Input: part model. Units: mm. Frame: model coordinates. Face numbers are marked on the shaded views. A direction names the side the tool comes from. Round coordinates to 2 decimals unless told otherwise and drop trailing zeros. Loops run counter-clockwise (first coordinate to the right, second up) from the corner with the lowest first, then second, coordinate; pieces in that order, holes last.
1) Section C-C, the plane y = 2.5. Return loops of the section in (x, z).
2) Section A-A, the plane z = 5.75. Return loops of the section in (x, y), and give its area (3 significant figures).
3) First-contact query: pin 1 (3 mm diameter, centred on y = -1.5, z = 10.5, fed in from +X); pin 2 (7.5 mm diameter, centred on x = 1, y = 8.5, fed in from +Z); pin 3 (1 mm diameter, centred on y = 13, z = 13, fed in from +X). Flat tips, straight axial feed; report the tip coordinate or a pass-through.
4) Draft query along X for the marked faces 1, 2, 3 and 4. Return one class per face: pulls with the +X half, pulls with the -X half, needs draft (parallel to the pull), parting line crosses it, or undercut.
5) Ray query, line 1 along Y through (x, z) = (-6.25, 11.25); line 2 along X through (y, z) = (-8.25, 2.15); line 3 along X through (y, z) = (-8.25, -1.2). Return the intervals inside material, ascending.
6) Section B-B, the plane x = 0. Return loops of the section in (y, z).
7) Access query for the marked faces 5, 6 and 7. Directions: +Z, -Z, +X, -X, +Y, -Y. A direction counts if a zero-diameter tool reaches every point of the face in a straight line with its end or side. Return the directions, or none.
from build123d import *

# Parameters (mm, degrees)
F4_DEPTH       = 13.5
F4_DEPTH_BACK  = 3
F5_R           = 4
F6_T           = -1.2
F7_W           = 6.6
F7_H           = 6
F8_DEPTH       = 13.75
F8_DEPTH_BACK  = 13.75
F3_W           = 8
F3_H           = 8.5
F9_DEPTH       = 4.5
F9_DEPTH_BACK  = 4.3
F11_START      = -6.5
F10_W          = 10.5
F10_H          = 18.4398862173
F11_DEPTH      = 11.4
F12_F1_R       = 4
F12_F2_R       = 4
F12_F3_R       = 4
F12_F4_R       = 4
F0_R           = 1.25
F13_DEPTH      = 7.9
F13_DEPTH_BACK = 7.1
F1_R           = 2.5
F14_DEPTH      = 1.8
F14_DEPTH_BACK = 4.3
F15_R          = 5
F17_DEPTH      = 16
F17_DEPTH_BACK = 16.1
F18_W          = 5.6
F18_H          = 3
F19_DEPTH      = 25
F19_DEPTH_BACK = 25


# Not quite as in the source:
# - a feature names something its author has since deleted; it is built from what else it names


with BuildPart() as f4:
    # F2 (on Top) → F4 (new body, two sides)
    with BuildSketch(Plane.XY) as f4_sk:
        with BuildLine():
            Line((2.6, 4.25), (2.6, 13.75))
            Line((2.6, 13.75), (-16, 13.75))
            Line((-16, 13.75), (-16, -13.75))
            Line((-16, -13.75), (2.6, -13.75))
            Line((2.6, -13.75), (2.6, -4.25))
            Line((2.6, -4.25), (-4.5505102572, -4.25))
            ThreePointArc((-4.5505102572, -4.25), (-8.769806787, -4.7695668459), (-10.3781091101, -0.8343697034))
            Line((-10.3781091101, -0.8343697034), (-9, 4.25))
            Line((-9, 4.25), (2.6, 4.25))
        make_face()
    extrude(amount=F4_DEPTH)
    extrude(f4_sk.sketch, amount=-F4_DEPTH_BACK)

    # F5
    f5_edges = [f4.edges().sort_by_distance(p)[0] for p in [
        (-16, 13.75, 5.25),
        (-16, -13.75, 5.25),
    ]]
    fillet(f5_edges, radius=F5_R)

    # F6
    f6_openings = [f4.faces().sort_by_distance(p)[0] for p in [
        (-4.7, 13.418005, 13.5),
        (2.6, 9, 5.25),
        (2.6, -9, 5.25),
        (-0.975255, -4.25, 5.25),
        (-3.2, 4.25, 5.25),
        (-8.769807, -4.769567, 5.25),
        (-9.689055, 1.707815, 5.25),
    ]]
    offset(amount=F6_T, openings=f6_openings)

    # F7 (on Front) → F8 (join, two sides)
    with BuildSketch(Plane.XZ) as f8_sk:
        with Locations((-0.7, 0)):
            Rectangle(F7_W, F7_H)
    extrude(amount=-F8_DEPTH)
    extrude(f8_sk.sketch, amount=F8_DEPTH_BACK)

    # F3 (on Top) → F9 (cut, two sides)
    with BuildSketch(Plane.XY) as f9_sk:
        with Locations((-1.4, 0)):
            Rectangle(F3_W, F3_H)
    extrude(amount=F9_DEPTH, mode=Mode.SUBTRACT)
    extrude(f9_sk.sketch, amount=-F9_DEPTH_BACK, mode=Mode.SUBTRACT)

    # F10 (on Right) → F11 (cut)
    with BuildSketch(Plane.YZ.offset(F11_START)):
        with Locations((2.5, 10.7199431086)):
            Rectangle(F10_W, F10_H)
    extrude(amount=-F11_DEPTH, mode=Mode.SUBTRACT)

    # F12: fillet of radius 4 on 4 edges, made by hand

    # F12_f1
    f12_f1_edges = [f4.edges().sort_by_distance(p)[0] for p in [
        (-4, -4.25, 0.6),
    ]]
    fillet(f12_f1_edges, radius=F12_F1_R)

    # F12_f2
    f12_f2_edges = [f4.edges().sort_by_distance(p)[0] for p in [
        (-4, 4.25, 0.6),
    ]]
    fillet(f12_f2_edges, radius=F12_F2_R)

    # F12_f3
    f12_f3_edges = [f4.edges().sort_by_distance(p)[0] for p in [
        (2.6, 4.25, 0),
    ]]
    fillet(f12_f3_edges, radius=F12_F3_R)

    # F12_f4
    f12_f4_edges = [f4.edges().sort_by_distance(p)[0] for p in [
        (2.6, -4.25, 0),
    ]]
    fillet(f12_f4_edges, radius=F12_F4_R)

    # F0 (on Top) → F13 (cut, two sides)
    with BuildSketch(Plane.XY) as f13_sk:
        with Locations((0, -8.25)):
            Circle(F0_R)
        with Locations((0, 8.25)):
            Circle(F0_R)
    extrude(amount=F13_DEPTH, mode=Mode.SUBTRACT)
    extrude(f13_sk.sketch, amount=-F13_DEPTH_BACK, mode=Mode.SUBTRACT)

    # F1 (on Top) → F14 (cut, two sides)
    with BuildSketch(Plane.XY) as f14_sk:
        with Locations((0, -8.25)):
            Circle(F1_R)
        with Locations((0, 8.25)):
            Circle(F1_R)
    extrude(amount=F14_DEPTH, mode=Mode.SUBTRACT)
    extrude(f14_sk.sketch, amount=-F14_DEPTH_BACK, mode=Mode.SUBTRACT)

    # F15
    f15_edges = [f4.edges().sort_by_distance(p)[0] for p in [
        (-4.55051, -4.25, -2.4),
        (-9, 4.25, -2.4),
    ]]
    fillet(f15_edges, radius=F15_R)

    # F16 (on Front) → F17 (cut, two sides)
    with BuildSketch(Plane.XZ) as f17_sk:
        Polygon((2.6, 1.8), (-4.0077234488, -6.074778159), (2.3954068281, -10.9375437775), (8.7053719483, -6.2603745918), align=None)
    extrude(amount=F17_DEPTH, mode=Mode.SUBTRACT)
    extrude(f17_sk.sketch, amount=-F17_DEPTH_BACK, mode=Mode.SUBTRACT)

    # F18 (on Front) → F19 (cut, two sides)
    with BuildSketch(Plane.XZ) as f19_sk:
        with Locations((-0.2, 13.5)):
            Rectangle(F18_W, F18_H)
    extrude(amount=F19_DEPTH, mode=Mode.SUBTRACT)
    extrude(f19_sk.sketch, amount=-F19_DEPTH_BACK, mode=Mode.SUBTRACT)


solid = f4.part
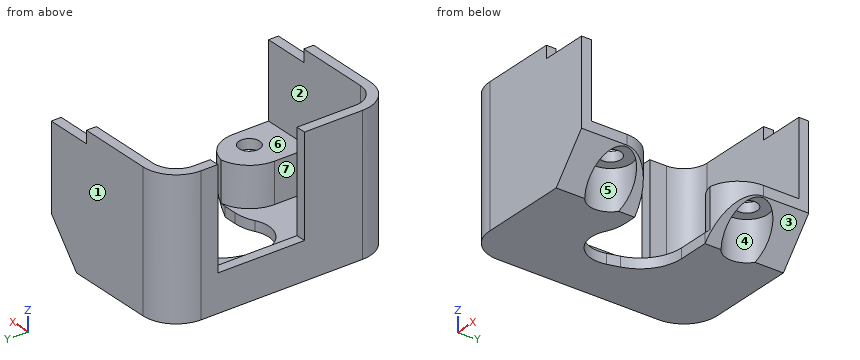
Final values:
1. outline: (-16, -3) - (-8.97, -3) - (-8.97, -1.8) - (-14.8, -1.8) - (-14.8, 1.5) - (-16, 1.5) - close
2. outline: (-16, -9.75) arc R4 ccw to (-12, -13.75) - (2.6, -13.75) - (2.6, -12.55) - (-12, -12.55) arc R2.8 cw to (-14.8, -9.75) - (-14.8, -2.75) - (-16, -2.75) - close; (-16, 7.75) - (-14.8, 7.75) - (-14.8, 9.75) arc R2.8 cw to (-12, 12.55) - (2.6, 12.55) - (2.6, 13.75) - (-12, 13.75) arc R4 ccw to (-16, 9.75) - close
2. area: 58.7 mm2
3. pin 1: stops at x = -14.8
3. pin 2: stops at z = 3
3. pin 3: stops at x = -3
4. face 1: needs draft
4. face 2: undercut
4. face 3: pulls with the +X half
4. face 4: undercut
5. line 1: y = -13.75 to -12.55, 12.55 to 13.75
5. line 2: x = -16 to -14.8, -4 to -1.25, 1.25 to 2.6
5. line 3: x = -16 to -14.8, -4 to -2.5
6. outline: (-13.75, -1.3) - (-10.75, -1.3) - (-10.75, 1.8) - (-9.5, 1.8) - (-9.5, 3) - (-12.55, 3) - (-12.55, 12) - (-13.75, 12) - close; (-7, 1.8) - (-5.75, 1.8) - (-5.75, -1.3) - (-4.5, -1.3) - (-4.5, 3) - (-7, 3) - close; (4.5, -1.3) - (5.75, -1.3) - (5.75, 1.8) - (7, 1.8) - (7, 3) - (4.5, 3) - close; (9.5, 1.8) - (10.75, 1.8) - (10.75, -1.3) - (13.75, -1.3) - (13.75, 12) - (12.55, 12) - (12.55, 3) - (9.5, 3) - close
7. face 5: -Z
7. face 6: +Z, +X
7. face 7: +Z
